Autodesk Inventor part; units mm, degrees
ref_plane "YZ Plane" through (0, 0, 0) normal (1, 0, 0) x (0, 1, 0)
ref_plane "XZ Plane" through (0, 0, 0) normal (0, 1, 0) x (-1, 0, 0)
ref_plane "XY Plane" through (0, 0, 0) normal (0, 0, 1) x (1, 0, 0)
ref_plane "Work Plane1" through (0, 0, 0) normal (0, 0, 1) x (1, 0, 0)
sketch "Sketch1" plane through (0, 0, 0) normal (0, 0, 1) x (1, 0, 0)
  arc A0 (-7.9352, -23.1681) -> (-8.7998, -28.0716) centre (-7.9352, -25.6961) ccw
  line L0 (-8.7998, -28.0716) -> (-27.4567, -41.1353)
  arc A1 (-34.704, -41.6104) -> (-27.4567, -41.1353) centre (-31.4718, -35.4013) ccw
  line L1 (-34.704, -41.6104) -> (-51.738, -32.743)
  arc A2 (-55.5058, -26.5339) -> (-51.738, -32.743) centre (-48.5058, -26.5339) ccw
  line L2 (-55.5058, -26.5339) -> (-55.5058, -22.4494)
  arc A3 (-49.7326, -15.5577) -> (-55.5058, -22.4494) centre (-48.5058, -22.4494) ccw
  line L3 (-49.7326, -15.5577) -> (-17.3058, -9.7854)
  line L4 (-17.3058, -9.7854) -> (-7.9352, -23.1681)
  line L5 (24.8783, -8.1523) -> (23.0703, -5.7559)
  line L6 (23.0703, -5.7559) -> (22.5789, -6.1)
  arc A4 (22.5789, -6.1) -> (17.1147, -5.1366) centre (19.7211, -6.3309) ccw
  line L7 (17.1147, -5.1366) -> (18.5334, -7.1626)
  circle A5 centre (19.7211, -6.3309) radius 1.45
  line L8 (18.5334, -7.1626) -> (19.2274, -8.1539)
  line L9 (19.2274, -8.1539) -> (-1.2514, -22.4933)
  line L10 (-1.2514, -22.4933) -> (-17.3116, 0.4431)
  line L11 (3.5665, 15.0622) -> (-17.3116, 0.4431)
  arc A6 (6.3584, 22.4292) -> (3.5665, 15.0622) centre (10.3734, 16.6951) ccw
  line L12 (6.3584, 22.4292) -> (14.6012, 28.2009)
  arc A7 (24.3503, 26.4818) -> (14.6012, 28.2009) centre (18.6163, 22.4668) ccw
  line L13 (24.3503, 26.4818) -> (36.2081, 9.5471)
  line L14 (36.2081, 9.5471) -> (39.0496, 11.5367)
  line L15 (39.0496, 11.5367) -> (25.5762, 30.7786)
  line L16 (25.5762, 30.7786) -> (31.5151, 34.937)
  line L17 (31.5151, 34.937) -> (47.862, 11.5912)
  line L18 (47.862, 11.5912) -> (41.9232, 7.4328)
  line L19 (41.9232, 7.4328) -> (43.6382, 4.9835)
  line L20 (43.6382, 4.9835) -> (58.5058, 15.3939)
  line L21 (58.5058, 15.3939) -> (40.3386, 41.3393)
  arc A8 (40.3386, 41.3393) -> (30.5895, 43.0583) centre (34.6046, 37.3243) ccw
  line L22 (30.5895, 43.0583) -> (-20.5271, 7.2661)
  arc A9 (-20.5271, 7.2661) -> (-23.5058, 1.8277) centre (-16.512, 1.532) ccw
  line L23 (-23.5058, 1.8277) -> (-20.3058, 1.8277)
  line L24 (-20.3058, 1.8277) -> (-20.3058, -7.2723)
  line L25 (-20.3058, -7.2723) -> (-72.9074, -16.6359)
  line L26 (-72.9074, -16.6359) -> (-72.9074, -24.0723)
  line L27 (-72.9074, -24.0723) -> (-58.5058, -24.0723)
  line L28 (-58.5058, -24.0723) -> (-58.5058, -28.3544)
  arc A10 (-58.5058, -28.3544) -> (-54.738, -34.5635) centre (-51.5058, -28.3544) ccw
  line L29 (-54.738, -34.5635) -> (-34.4745, -45.112)
  arc A11 (-34.4745, -45.112) -> (-27.2272, -44.637) centre (-31.2423, -38.9029) ccw
  line L30 (-27.2272, -44.637) -> (23.0703, -9.4182)
  arc A12 (27.0854, -8.1523) -> (23.0703, -9.4182) centre (27.0854, -15.1523) ccw
  line L31 (24.8783, -8.1523) -> (27.0854, -8.1523)
  circle A13 centre (-7.9352, -25.6961) radius 1.45
  circle A14 centre (25.9387, 36.6719) radius 1.45
  line L32 (24.8783, -8.1523) -> (35.6777, -8.1523)
  line L33 (35.6777, -8.1523) -> (35.6777, 3.8477) construction
  line L34 (35.6777, 3.8477) -> (95.6777, 3.8477) construction
  line L35 (95.6777, 3.8477) -> (95.6777, 15.3939)
  line L36 (95.6777, 15.3939) -> (58.5058, 15.3939)
  line L37 (58.5058, 15.3939) -> (43.6382, 4.9835)
  line L38 (43.6382, 4.9835) -> (39.0496, 11.5367)
  line L39 (39.0496, 11.5367) -> (32.6777, 7.0751)
  line L40 (32.6777, 7.0751) -> (32.6777, 0.9712)
  line L41 (32.6777, 0.9712) -> (23.0703, -5.7559)
  line L42 (23.0703, -5.7559) -> (24.8783, -8.1523)
  line L43 (24.9804, -8.4763) -> (23.0739, -5.7534)
  line L44 (23.0739, -5.7534) -> (32.6777, 0.9712)
  line L45 (32.6777, 0.9712) -> (32.6777, 7.0751)
  line L46 (32.6777, 7.0751) -> (39.0496, 11.5367)
  line L47 (39.0496, 11.5367) -> (43.6382, 4.9835)
  line L48 (43.6382, 4.9835) -> (58.5058, 15.3939)
extrude "Extrusion1" add sketch "Sketch1" along normal blind 1 contours A0 L0 A1 L1 A2 L2 A3 L3 L4 | A5 | L43 A12 L30 A11 L29 A10 L28 L27 L26 L25 L24 L23 A9 L22 A8 L21 L20 L19 L18 L17 L16 L15 L14 L13 A7 L12 A6 L11 L10 L9 L8 L7 A4 L6 L5 | L5 L41 L43 | L6 A4 L7 L8 L9 L10 L11 A6 L12 A7 L13 L39 L40 L41 | L15 L16 L17 L18 L38 | A13 | A14
sketch "Sketch2" plane through (0, 0, 1) normal (0, 0, 1) x (1, 0, 0)
  arc A0 (24.9804, -8.4763) -> (23.0703, -9.4182) centre (27.0854, -15.1523) ccw
  line L0 (24.9804, -8.4763) -> (23.0739, -5.7534)
  line L1 (23.0739, -5.7534) -> (32.6777, 0.9712)
  line L2 (32.6777, 0.9712) -> (32.6777, 7.0751)
  line L3 (32.6777, 7.0751) -> (39.0496, 11.5367)
  line L4 (39.0496, 11.5367) -> (43.6382, 4.9835)
  line L5 (43.6382, 4.9835) -> (58.5058, 15.3939)
  line L6 (58.5058, 15.3939) -> (40.3386, 41.3393)
  arc A1 (40.3386, 41.3393) -> (30.5895, 43.0583) centre (34.6046, 37.3243) ccw
  line L7 (30.5895, 43.0583) -> (-20.5271, 7.2661)
  arc A2 (-20.5271, 7.2661) -> (-23.5058, 1.8277) centre (-16.512, 1.532) ccw
  line L8 (-23.5058, 1.8277) -> (-20.3058, 1.8277)
  line L9 (-20.3058, 1.8277) -> (-20.3058, -7.2723)
  line L10 (-20.3058, -7.2723) -> (-72.9074, -16.6359)
  line L11 (-72.9074, -16.6359) -> (-72.9074, -24.0723)
  line L12 (-72.9074, -24.0723) -> (-58.5058, -24.0723)
  line L13 (-58.5058, -24.0723) -> (-58.5058, -28.3544)
  arc A3 (-58.5058, -28.3544) -> (-54.738, -34.5635) centre (-51.5058, -28.3544) ccw
  line L14 (-54.738, -34.5635) -> (-34.4745, -45.112)
  arc A4 (-34.4745, -45.112) -> (-27.2272, -44.637) centre (-31.2423, -38.9029) ccw
  line L15 (-27.2272, -44.637) -> (23.0703, -9.4182)
  circle A5 centre (25.9387, 36.6719) radius 1.45
  circle A6 centre (-7.9352, -25.6961) radius 1.45
  circle A7 centre (19.7211, -6.3309) radius 1.45
  point P0 (0, 0)
extrude "Extrusion2" cut sketch "Sketch2" against normal blind 1 contours A5 | A6 | A7
sketch "Sketch3" plane through (0, 0, 1) normal (0, 0, 1) x (1, 0, 0)
  line L0 (47.862, 11.5912) -> (31.5151, 34.937)
  line L1 (31.5151, 34.937) -> (25.5762, 30.7786)
  line L2 (41.9232, 7.4328) -> (25.5762, 30.7786)
  line L3 (47.862, 11.5912) -> (41.9232, 7.4328)
  line L4 (31.6379, 35.6334) -> (48.5584, 11.4684)
  line L5 (48.5584, 11.4684) -> (41.8004, 6.7364)
  line L6 (41.8004, 6.7364) -> (24.8799, 30.9014)
  line L7 (24.8799, 30.9014) -> (31.6379, 35.6334)
  point P0 (0, 0)
  dimension "d4" = 0.5
extrude "Extrusion3" cut sketch "Sketch3" against normal through all contours L3 L2 L1 L0 | L4 L5 L6 L7
properties part number "cellSTORM_inverted_opticsmodule_lid"
Here's how the part is built. I have some questions about the finished solid (model axes, mm). A direction names the side the tool comes from. Give positions to 0.01 mm unless a question says otherwise; leave off trailing zeros. Loops run counter-clockwise (first coordinate to the right, second up) from the corner with the lowest first, then second, coordinate; pieces in that order, holes last. Notation, with made-up numbers: (37, 23.5) -> (90, 23.5) arc R24 cw to (90, 38.5) -> close; hole circle Ø8 at (18.25, 51). An arc over 180 degrees is marked (long way). Use one line per item in the form item = value. Start each with the question number.
1) Thinking about a two-plate mould opening in Y: for faces 4 (the face through (31.856, 20.938, 0.507)), 5 (the face through (49.549, 28.185, 0.493)), 6 (the face through (-57.462, -32.031, 0.493)), which applies, +Y half, -Y half, draft (parallel to the pull), parting line (faces both ways), or undercut?
2) Imagine slicing it at C-C (x = 15). Please give me the cut outline in (y, z).
3) For P1, Ø0.5, axis at x = -68, z = 0.5, coming from the -Y side, with a flat end and sliding along its axis, tell me the tip position at first contact or that it passes through.
4) Please list where these lines run through material, in increasing order: line 1 along X through (y, z) = (35.5, 0.55); line 2 along Y through (x, z) = (47, 0.7); line 3 along Y through (x, z) = (30.5, 0.55).
5) Imagine slicing it at A-A (y = 21.5). Please give me the cut outline in (x, z), then the cut area to 3 significant figures.
6) Imagine slicing it at D-D (y = 33.5). Please give me the cut outline in (x, z), then the cut area to 3 significant figures.
7) Imagine slicing it at B-B (z = 0.35). Count the separate pieces of the cut face and the enclosed holes in it, then the cut area to 3 significant figures.
8) Which directions (+Z, -Z, +X, -X, +Y, -Y) give clear straight access to the entire face, cutting with the end or side of a thin tool? Please do faces 1 (the face through (27.943, -2.344, 0.493)), 2 (the face through (39.98, 23.72, 0.51)), 3 (the face through (50.968, 10.116, 0.493)).
Check values:
q1.face_4 = undercut
q1.face_5 = +Y half
q1.face_6 = -Y half
q2.outline = (-15.07, 0) -> (32.14, 0) -> (32.14, 1) -> (-15.07, 1) -> close
q3.P1 = -24.07
q4.line_1 = 19.8 to 25.08, 26.79 to 31.45, 31.73 to 44.43
q4.line_2 = 7.34 to 10.38, 13.69 to 31.83
q4.line_3 = -0.55 to 22.88, 34.84 to 43
q5.outline = (-0.2, 0) -> (31.46, 0) -> (31.46, 1) -> (-0.2, 1) -> close; (41.53, 0) -> (54.23, 0) -> (54.23, 1) -> (41.53, 1) -> close
q5.area = 44.4 mm^2
q6.outline = (16.94, 0) -> (28.59, 0) -> (28.59, 1) -> (16.94, 1) -> close; (33.13, 0) -> (45.83, 0) -> (45.83, 1) -> (33.13, 1) -> close
q6.area = 24.3 mm^2
q7.separate_pieces = 1
q7.enclosed_holes = 3
q7.area = 4,090 mm^2
q8.face_1 = +Z, -Z, +X
q8.face_2 = +Z, -Z
q8.face_3 = +Z, -Z, +X, -Y
